from build123d import *

# Parameters (mm, degrees)
BOSS_EXTRUDE1_DEPTH     = 1.3
BOSS_EXTRUDE2_DEPTH     = 1.76
CIRPATTERN1_COUNT       = 4
CUT_EXTRUDE2_DEPTH      = 15.794267561
CUT_EXTRUDE2_DEPTH_BACK = 15.794267561
CUT_EXTRUDE3_DEPTH      = 15.794267603
CUT_EXTRUDE3_DEPTH_BACK = 15.794267603
SKETCH8_W               = 3.75
SKETCH8_H               = 7
FILLET1_R               = 0.2


with BuildPart() as part:
    # Sketch1 → Boss-Extrude1 (new body)
    with BuildSketch(Plane(origin=(0, 0, 0), x_dir=(1, 0, 0), z_dir=(0, 1, 0))):
        with BuildLine():
            Line((-0.730769231, 7.71160656), (5.548073923, 7.71160656))
            ThreePointArc((5.548073923, 7.71160656), (8.281459084, 4.65482926), (9.47185179, 0.730769231))
            Line((9.47185179, 0.730769231), (7.71160656, 0.730769231))
            Line((7.71160656, 0.730769231), (7.71160656, -5.548073923))
            ThreePointArc((7.71160656, -5.548073923), (4.65482926, -8.281459084), (0.730769231, -9.47185179))
            Line((0.730769231, -9.47185179), (0.730769231, -7.71160656))
            Line((0.730769231, -7.71160656), (-5.548073923, -7.71160656))
            ThreePointArc((-5.548073923, -7.71160656), (-8.281459084, -4.65482926), (-9.47185179, -0.730769231))
            Line((-9.47185179, -0.730769231), (-7.71160656, -0.730769231))
            Line((-7.71160656, -0.730769231), (-7.71160656, 5.548073923))
            ThreePointArc((-7.71160656, 5.548073923), (-4.65482926, 8.281459084), (-0.730769231, 9.47185179))
            Line((-0.730769231, 9.47185179), (-0.730769231, 7.71160656))
        make_face()
    extrude(amount=BOSS_EXTRUDE1_DEPTH)

    # Sketch2 → Boss-Extrude2 (add)
    with BuildSketch(Plane(origin=(0, 0, -7.71160656), x_dir=(-1, 0, 0), z_dir=(0, 0, -1))):
        with BuildLine():
            Line((-0.730769231, 6.28), (-0.730769231, 1.3))
            ThreePointArc((-0.730769231, 1.3), (-0.24725105, 0.372025447), (0.730769231, 0))
            Line((0.730769231, 0), (0.730769231, 1.3))
            ThreePointArc((0.730769231, 1.3), (0.26383811, 1.463095229), (0, 1.881442187))
            Line((0, 1.881442187), (0, 5.549230769))
            Line((0, 5.549230769), (-0.730769231, 6.28))
        make_face()
    boss_extrude2 = extrude(amount=BOSS_EXTRUDE2_DEPTH)

    # CirPattern1: Boss-Extrude2 ×4 about axis
    cirpattern1_axis = Axis((0, 0, 0), (0, 1, 0))
    for i in range(1, CIRPATTERN1_COUNT):
        add(boss_extrude2.rotate(cirpattern1_axis, i * 360 / CIRPATTERN1_COUNT))

    # Sketch6 → Cut-Extrude2 (cut, two sides: drawn at the far end of the back side and taken through both)
    with BuildSketch(Plane(origin=(0, 0, 0), x_dir=(0, 0, -1), z_dir=(1, 0, 0)).offset(-CUT_EXTRUDE2_DEPTH_BACK)):
        with BuildLine():
            Line((-7.71160656, 6.28), (-9.47160656, 6.28))
            Line((-9.47160656, 6.28), (-9.47185179, 1.3))
            ThreePointArc((-9.47185179, 1.3), (-9.018842539, 3.940968727), (-7.71160656, 6.28))
        make_face()
        with BuildLine():
            Line((7.71160656, 6.28), (9.47160656, 6.28))
            Line((9.47160656, 6.28), (9.47185179, 1.3))
            ThreePointArc((9.47185179, 1.3), (9.018842539, 3.940968727), (7.71160656, 6.28))
        make_face()
    extrude(amount=CUT_EXTRUDE2_DEPTH + CUT_EXTRUDE2_DEPTH_BACK, mode=Mode.SUBTRACT)

    # Sketch7 → Cut-Extrude3 (cut, two sides: drawn at the far end of the back side and taken through both)
    with BuildSketch(Plane.XY.offset(-CUT_EXTRUDE3_DEPTH_BACK)):
        with BuildLine():
            Line((-9.47160656, 6.28), (-7.71160656, 6.28))
            ThreePointArc((-7.71160656, 6.28), (-9.018842539, 3.940968727), (-9.47185179, 1.3))
            Line((-9.47185179, 1.3), (-9.47160656, 6.28))
        make_face()
        with BuildLine():
            Line((9.47160656, 6.28), (7.71160656, 6.28))
            ThreePointArc((7.71160656, 6.28), (9.018842539, 3.940968727), (9.47185179, 1.3))
            Line((9.47185179, 1.3), (9.47160656, 6.28))
        make_face()
    extrude(amount=CUT_EXTRUDE3_DEPTH + CUT_EXTRUDE3_DEPTH_BACK, mode=Mode.SUBTRACT)

    # Sketch8 → Revolve1 (revolve)
    with BuildSketch(Plane.XY):
        with Locations((1.875, 4.8)):
            Rectangle(SKETCH8_W, SKETCH8_H)
    revolve(axis=Axis((0, 1.3, 0), (0, 1, 0)))

    # Fillet1
    fillet1_edges = [part.edges().sort_by_distance(p)[0] for p in [
        (-3.75, 1.3, 0),
    ]]
    fillet(fillet1_edges, radius=FILLET1_R)

    # Sketch10 → M6 Tapped Hole1 (revolve, cut)
    with BuildSketch(Plane(origin=(0, 0, 0), x_dir=(0, 0, -1), z_dir=(1, 0, 0))):
        Polygon((0, 0), (0, 8.3), (3.025, 8.3), (2.5, 7.775), (2.5, 0.525), (3.025, 0), align=None)
    revolve(axis=Axis((0, -6.35, 0), (0, 1, 0)), mode=Mode.SUBTRACT)


solid = part.part
Geometry check sheet. Reference: the model listing, model coordinates, mm. A direction names the side the tool comes from. Round coordinates to 2 decimals unless told otherwise and drop trailing zeros. Order: outer loops, then holes, each group sorted by start corner. A loop starts at its lowest first (then second) coordinate and runs counter-clockwise, first axis right, second up. Notation, with made-up numbers: M 54.5,17 L 112.5,17 A32 ccw 112.5,44 Z; hole C 39.25,0.5 d4. An arc over 180 degrees is marked long. Answer in a Markdown table with one row per item. Add a question column.
Item 1: Material ranges on L1, parallel to Y at x = -1.75, z = -8.25; L2, parallel to X at y = 2.75, z = 8.75; L3, parallel to Z at x = 0.5, y = 1.75, recorded low to high. Write a range as [from, to].
Item 2: Sectioned sample at C-C, the plane y = 7. Enter the section's corners in (x, z), plus the area to 3 significant figures.
Item 3: Depth check by flat-ended pin: pin 1 Ø1.6 at (x, y) = (0, 4.5) entering from +Z; pin 2 Ø0.7 at (x, y) = (1.5, 0.5) entering from -Z; pin 3 Ø3 at (y, z) = (6.5, -3.5) entering from +X; pin 4 Ø4 at (x, z) = (0, 0) entering from +Y. Enter the tip coordinate at first touch or a pass-through.
Item 4: Sectioned sample at B-B, the plane y = 3. Enter the section's corners in (x, z), plus the area to 3 significant figures.
Item 5: Sectioned sample at A-A, the plane y = 4. Enter the section's corners in (x, z), plus the area to 3 significant figures.
Item 6: Set-up check for faces 5 (the face through (-8, 3, -0.731)), 6 (the face through (-8.579, 0.382, -0.258)), 7 (the face through (-3.746, 4.948, -0.165)), 8 (the face through (8.579, 0.382, 0.258)): record each of +Z, -Z, +X, -X, +Y, -Y from which the full face is reachable in a straight line by a thin tool's end or side.
Item 7: Draft check along Z on faces 1 (the face through (-8.25, 0.64, 4.71)), 2 (the face through (-0.3, 3.8, 7.712)), 3 (the face through (0, 3, -8)), 4 (the face through (8, 3, 0)). Enter one of: released by +Z, released by -Z, zero draft, split by the parting line, or undercut.
Item 8: Sectioned sample at D-D, the plane z = -4.25. Enter the section's corners in (x, y).
Filled in:
| question | item | result |
|---|---|---|
| 1 | L1 | y = [0, 1.3] |
| 1 | L2 | x = [-0.73, 0] |
| 1 | L3 | z = [-9.46, -7.71], [-3.72, -2.45], [2.45, 3.72] |
| 2 | outline | C 0,0 d7.5; hole C 0,0 d5 |
| 2 | area | 24.5 mm² |
| 3 | pin 1 | stops at z = 9.1 |
| 3 | pin 2 | stops at z = -7.71 |
| 3 | pin 3 | stops at x = 3.17 |
| 3 | pin 4 | passes through |
| 4 | outline | M -9.29,-0.73 L -7.71,-0.73 L -7.71,0 L -9.29,0 Z; C 0,0 d7.5; M -0.73,7.71 L 0,7.71 L 0,9.29 L -0.73,9.29 Z; M 0,-9.29 L 0.73,-9.29 L 0.73,-7.71 L 0,-7.71 Z; M 7.71,0 L 9.29,0 L 9.29,0.73 L 7.71,0.73 Z; hole C 0,0 d5 |
| 4 | area | 29.1 mm² |
| 5 | outline | M -9,-0.73 L -7.71,-0.73 L -7.71,0 L -9,0 Z; C 0,0 d7.5; M -0.73,7.71 L 0,7.71 L 0,9 L -0.73,9 Z; M 0,-9 L 0.73,-9 L 0.73,-7.71 L 0,-7.71 Z; M 7.71,0 L 9,0 L 9,0.73 L 7.71,0.73 Z; hole C 0,0 d5 |
| 5 | area | 28.3 mm² |
| 6 | face 5 | -Z, -X, +Y, -Y |
| 6 | face 6 | -Z, -X, -Y |
| 6 | face 7 | +Y |
| 6 | face 8 | +Z, +X, -Y |
| 7 | face 1 | released by +Z |
| 7 | face 2 | undercut |
| 7 | face 3 | zero draft |
| 7 | face 4 | released by -Z |
| 8 | outline | M -7.71,0 L 8.5,0 L 8.5,1.3 L -7.71,1.3 Z |
